Design review of the part built by this model. Coordinates are the model's own, in mm. A direction names the side the tool comes from. Give positions to 0.01 mm unless a question says otherwise; leave off trailing zeros. Order: outer loops, then holes, each group sorted by start corner. A loop starts at its lowest first (then second) coordinate and runs counter-clockwise, first axis right, second up. Notation, with made-up numbers: (6, 84.25) -> (32, 84.25) arc R32 ccw to (32, 119.25) -> close; hole circle Ø11 at (27.25, 39). An arc over 180 degrees is marked (long way). One line per item, written item: value. Start each with the question number.
1) Tool access review of faces 4 (the face through (224.051, 242.865, 22.25)), 5 (the face through (203, 225.191, 13)), 6 (the face through (220, 235, 20)): name each direction out of +Z, -Z, +X, -X, +Y, -Y from which nothing blocks a thin tool from reaching the whole face with its end or side.
2) For pin 1 (6 mm diameter, centred on y = 244, z = 48.5, fed in from -X); pin 2 (10 mm diameter, centred on y = 218.5, z = 30, fed in from +X); pin 3 (1 mm diameter, centred on x = 206, y = 228, fed in from +Z), all flat-tipped, find the tip position at first contact; note any pin that passes through.
3) The part is to be moulded in two halves that separate along Y. For faces 1 (the face through (214, 222, 0)), 2 (the face through (216.82, 231.53, 12.11)), 3 (the face through (220.124, 249.749, 31.707)), say which applies: released by +Y, released by -Y, zero draft, split by the parting line, or undercut.
4) Consider section A-A (z = 47). State the section outline as (x, y) points.
5) Wall thickness on line 1 along Y through (x, z) = (212.5, 19.5); line 2 along Z through (x, y) = (200.5, 214.5); line 3 along Z through (x, y) = (215, 230.5): over which ranges is each line inside the solid? List them lowest first. Write a range as from..to.
from build123d import *

# Parameters (mm, degrees)
SKETCH1_W                       = 28
SKETCH1_H                       = 37
BOSS_EXTRUDE1_DEPTH             = 4
EXTRUDE_THIN1_DEPTH             = 60
BOSS_EXTRUDE2_DEPTH             = 18.5
BOSS_EXTRUDE2_DEPTH_BACK        = 3
SKETCH5_R                       = 12
BOSS_EXTRUDE4_REACH             = 356.551
BOSS_EXTRUDE4_DIRECTION_2_DEPTH = 19
CUT_EXTRUDE2_DEPTH              = 363.265046463
CHAMFER1_START                  = 52.77449686
CHAMFER1_DEPTH                  = 8.045724116
FILLET1_R                       = 5
SKETCH12_R                      = 2
CUT_EXTRUDE3_DEPTH              = 11
CHAMFER3_SIZE                   = 1
CHAMFER3_SIZE2                  = 0.577350269
RIB2_START                      = -1.5
RIB2_DEPTH                      = 3
SKETCH13_R                      = 1.5
CUT_EXTRUDE6_DEPTH              = 11
FILLET2_R                       = 5
CUT_REVOLVE_START               = 202.331523811
CUT_REVOLVE_3_OUTLINE_R         = 9.25
CUT_REVOLVE_3_DEPTH             = 25.093721499


with BuildPart() as part:
    # Sketch1 → Boss-Extrude1 (new body)
    with BuildSketch(Plane.XY):
        with Locations((214.317546036, 222.190706617)):
            Rectangle(SKETCH1_W, SKETCH1_H)
    extrude(amount=BOSS_EXTRUDE1_DEPTH)

    # Sketch4 → Extrude-Thin1 (add, along a direction that is not the sketch's normal)
    with BuildSketch(Plane.XY.offset(4)):
        Polygon((214.894152277, 240.690706617), (228.317546036, 232.940706617), (224.317546036, 226.012503387), (210.894152277, 233.762503387), align=None)
    extrude(amount=EXTRUDE_THIN1_DEPTH, dir=(0.22699524986977232, 0.3931673058512374, 0.8910065241883693))

    # Sketch5 → Boss-Extrude2 (add, two sides: drawn at the far end of the back side and taken through both)
    with BuildSketch(Plane(origin=(0, 222.190706617, 0), x_dir=(-1, 0, 0), z_dir=(0, -1, 0)).offset(-BOSS_EXTRUDE2_DEPTH_BACK)):
        with BuildLine():
            Line((-191.578997844, -17.916678927), (-200.317546036, 0))
            Line((-200.317546036, 0), (-216.317546036, 0))
            Line((-216.317546036, 0), (-216.317546036, -4))
            Line((-216.317546036, -4), (-214.306389256, -24.35692569))
            ThreePointArc((-214.306389256, -24.35692569), (-205.636142491, -11.631721126), (-191.578997844, -17.916678927))
        make_face()
        with Locations((-202.3645264, -23.177132689)):
            Circle(SKETCH5_R)
    extrude(amount=BOSS_EXTRUDE2_DEPTH + BOSS_EXTRUDE2_DEPTH_BACK)

    # Boss-Extrude4: up to this face of the body (flat: up to its plane)
    boss_extrude4_end = Plane(part.part.faces().sort_by_distance((228.317546036, 222.190706617, 2))[0])
    # Sketch7 → Boss-Extrude4 (add, up to the picked face)
    with BuildSketch(Plane(origin=(70.371874774, -40.629220844, 0), x_dir=(0, 0, -1), z_dir=(0.8660254037844386, -0.5, 0)), mode=Mode.PRIVATE) as boss_extrude4_sk1:
        Polygon((-4, 315.891342524), (-19.700884044, 315.891342524), (-4, 307.891342524), align=None)
    boss_extrude4_tool1 = split(extrude(boss_extrude4_sk1.sketch, amount=BOSS_EXTRUDE4_REACH, mode=Mode.PRIVATE), bisect_by=boss_extrude4_end, keep=Keep.BOTH, mode=Mode.PRIVATE)
    add(boss_extrude4_tool1.solids().sort_by(Axis((226.984213, 230.631306, 9.233628), (0.8660254037844386, -0.5, 0)))[0])

    # Sketch7 → Boss-Extrude4 direction 2 (add)
    with BuildSketch(Plane(origin=(70.371874774, -40.629220844, 0), x_dir=(0, 0, -1), z_dir=(0.8660254037844386, -0.5, 0))):
        Polygon((-4, 315.891342524), (-19.700884044, 315.891342524), (-4, 307.891342524), align=None)
    extrude(amount=-BOSS_EXTRUDE4_DIRECTION_2_DEPTH)

    # Sketch8 → Cut-Extrude2 (cut, through all)
    with BuildSketch(Plane(origin=(0, 0, 4), x_dir=(-1, 0, 0), z_dir=(0, 0, -1))):
        Polygon((-214.894152277, 240.690706617), (-210.852700393, 240.690706617), (-211.863063364, 242.440706617), align=None)
    extrude(amount=-CUT_EXTRUDE2_DEPTH, mode=Mode.SUBTRACT)

    # Chamfer1: read off the stored shape, not the designer's step
    # Chamfer1 outline → Chamfer1 (cut)
    with BuildSketch(Plane(origin=(0, 0, 0), x_dir=(0.5316074109578968, 0.7735134037427047, 0.3450660441785277), z_dir=(0.8469908857919558, -0.48548982616312697, -0.21657808771308096)).offset(CHAMFER1_START)):
        Polygon((307.114108085, -80.169957731), (294.178723025, -92.183926772), (299.729695769, -94.190354162), align=None)
    extrude(amount=CHAMFER1_DEPTH, mode=Mode.SUBTRACT)

    # Fillet1
    # the kernel refuses this fillet: 5 mm, written as the material it adds along each edge
    with BuildSketch(Plane(origin=(197.228839574, 250.889779662, 4), x_dir=(0.49999999999999944, 0.8660254037844389, 0), z_dir=(0.866025403784439, -0.4999999999999995, 0))) as fillet1_piece_1_section:
        with BuildLine():
            CenterArc((FILLET1_R * 1.63185168713, FILLET1_R), FILLET1_R, 153, 117)
            Line((FILLET1_R * 0.74084516294, FILLET1_R * 1.45399049974), (0, 0))
            Line((0, 0), (FILLET1_R * 1.63185168713, 0))
        make_face()
    fillet1_piece_1 = extrude(amount=56.296292178, mode=Mode.PRIVATE)
    fillet1_piece_1 = split(fillet1_piece_1, bisect_by=Plane(origin=(228.317546036, 250.889779662, 4), z_dir=(-1, 0, 0)), keep=Keep.TOP, mode=Mode.PRIVATE)
    fillet1_piece_1 = split(fillet1_piece_1, bisect_by=Plane(origin=(197.228839574, 240.690706617, 4), z_dir=(0, -1, 0)), keep=Keep.TOP, mode=Mode.PRIVATE)
    add(fillet1_piece_1)

    # Sketch12 → Cut-Extrude3 (cut)
    with BuildSketch(Plane.XY.offset(4)):
        with Locations((205.117546036, 231.690706617)):
            Circle(SKETCH12_R)
        with Locations((223.517546036, 212.690706617)):
            Circle(SKETCH12_R)
    extrude(amount=-CUT_EXTRUDE3_DEPTH, mode=Mode.SUBTRACT)

    # Chamfer3
    chamfer3_edges = [part.edges().sort_by_distance(p)[0] for p in [
        (203.117546036, 231.690706617, 4),
        (221.517546036, 212.690706617, 4),
    ]]
    chamfer3_side = [part.faces().sort_by_distance(p)[0] for p in [
        (208.956042358, 238.333607157, 4),
    ]]
    chamfer(chamfer3_edges, length=CHAMFER3_SIZE, length2=CHAMFER3_SIZE2, reference=chamfer3_side[0])

    # Rib2: read off the stored shape, not the designer's step
    # Rib2 outline → Rib2 (add)
    with BuildSketch(Plane(origin=(63.660177895, -36.754220844, 0), x_dir=(-0.49999999999999845, -0.8660254037844396, 0), z_dir=(-0.8660254037844396, 0.49999999999999845, 0)).offset(RIB2_START)):
        Polygon((-301.043749716, 4), (-311.043749716, 20), (-316.043749716, 20), (-307.891342524, 4), align=None)
    extrude(amount=RIB2_DEPTH)

    # Sketch13 → Cut-Extrude6 (cut)
    with BuildSketch(Plane(origin=(124.582886752, 215.783889609, -126.956302744), x_dir=(0.8952803155791154, -0.38397537070557247, 0.2259116447376676), z_dir=(0.44550326209418484, 0.7716342848848018, -0.45399049973954403))):
        with Locations(Location((122.316663554, -176.73795859, 0), (0, 0, 270))):
            Circle(SKETCH13_R)
        with Locations(Location((112.935440602, -140.94700085, 0), (0, 0, 270))):
            Circle(SKETCH13_R)
    extrude(amount=-CUT_EXTRUDE6_DEPTH, mode=Mode.SUBTRACT)

    # Fillet2
    fillet2_edges = [part.edges().sort_by_distance(p)[0] for p in [
        (239.937261028, 253.066643353, 57.460391451),
        (226.51386727, 260.816643353, 57.460391451),
    ]]
    fillet(fillet2_edges, radius=FILLET2_R)

    # Chamfer4: read off the stored shape, not the designer's step
    # Chamfer4: loft between two sections, ruled curve by curve
    chamfer4_from = [
        Edge.make_three_point_arc((233.094750309, 254.144111481, 56.022204084), (231.428373697, 255.374841148, 56.47881494), (230.517297529, 254.821743623, 54.644687533)),
        Edge.make_three_point_arc((230.517297529, 254.821743623, 54.644687533), (232.183674141, 253.591013956, 54.188076677), (233.094750309, 254.144111481, 56.022204084)),
    ]
    chamfer4_to = [
        Edge.make_three_point_arc((233.195805822, 252.340022177, 57.460391452), (230.246651896, 254.518167985, 58.268501508), (228.634228967, 253.539295786, 55.022462165)),
        Edge.make_three_point_arc((228.634228967, 253.539295786, 55.022462165), (231.583382893, 251.361149979, 54.214352108), (233.195805822, 252.340022177, 57.460391452)),
    ]
    chamfer4 = Solid(Shell([*[Face.make_surface_from_curves(chamfer4_from[k], chamfer4_to[k]) for k in range(2)], Face(Wire(chamfer4_from)), Face(Wire(chamfer4_to))]))
    add(chamfer4, mode=Mode.SUBTRACT)

    # Chamfer4 2: loft between two sections, ruled curve by curve
    chamfer4_2_from = [
        Edge.make_three_point_arc((223.407199674, 240.696376934, 23.659041313), (222.064279201, 240.511700292, 22.027336946), (223.407199674, 239.175097537, 21.073367514)),
        Edge.make_three_point_arc((223.407199674, 239.175097537, 21.073367514), (224.750120147, 239.359774179, 22.705071881), (223.407199674, 240.696376934, 23.659041313)),
    ]
    chamfer4_2_to = [
        Edge.make_three_point_arc((222.51619315, 239.738649078, 25.562248622), (220.139492014, 239.411808289, 22.674457648), (222.51619315, 237.046288254, 20.986122204)),
        Edge.make_three_point_arc((222.51619315, 237.046288254, 20.986122204), (224.892894286, 237.373129042, 23.873913178), (222.51619315, 239.738649078, 25.562248622)),
    ]
    chamfer4_2 = Solid(Shell([*[Face.make_surface_from_curves(chamfer4_2_from[k], chamfer4_2_to[k]) for k in range(2)], Face(Wire(chamfer4_2_from)), Face(Wire(chamfer4_2_to))]))
    add(chamfer4_2, mode=Mode.SUBTRACT)

    # 切除-旋转3: read off the stored shape, not the designer's step
    # 切除-旋转3 outline → 切除-旋转3 (cut)
    with BuildSketch(Plane(origin=(0, 0, 0), x_dir=(1, 0, 0), z_dir=(0, 0.984807753012207, 0.173648177666937)).offset(CUT_REVOLVE_START)):
        with Locations((202.3645264, 16.278935867)):
            Circle(CUT_REVOLVE_3_OUTLINE_R)
    extrude(amount=CUT_REVOLVE_3_DEPTH, mode=Mode.SUBTRACT)


solid = part.part
Checked values:
1. face 4: none
1. face 5: +Z, -X
1. face 6: +Z, -X, -Y
2. pin 1: stops at x = 232.48
2. pin 2: stops at x = 214.23
2. pin 3: stops at z = 4
3. face 1: zero draft
3. face 2: undercut
3. face 3: released by +Y
4. outline: (221.85, 252.74) -> (235.27, 244.99) -> (239.27, 251.91) -> (225.85, 259.66) -> close
5. line 1: y = 203.69..225.19
5. line 2: z = 0..12.09, 30.49..35.03
5. line 3: z = 0..4
